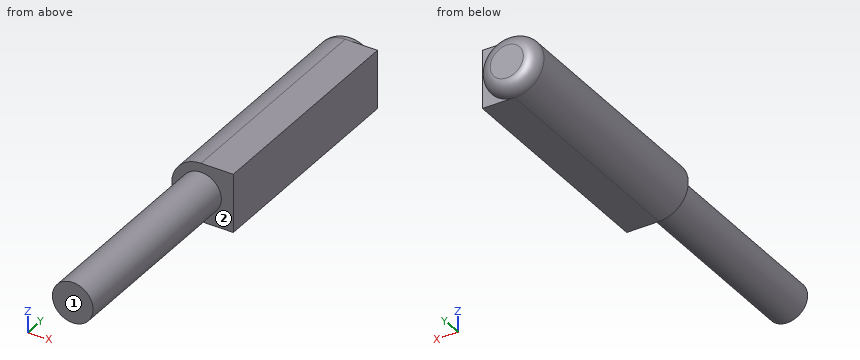
```python
from build123d import *

# Parameters (mm, degrees)
F0_R     = 11.5
F2_DEPTH = 95
F1_R     = 8
F3_DEPTH = 80
F4_R     = 5
F5_W     = 90
F5_H     = 23
F6_DEPTH = 12.7


with BuildPart() as f2:
    # F0 (on Front) → F2 (new body)
    with BuildSketch(Plane.XZ):
        Circle(F0_R)
    extrude(amount=-F2_DEPTH)

    # F1 (on Front) → F3 (join)
    with BuildSketch(Plane.XZ):
        Circle(F1_R)
    extrude(amount=F3_DEPTH)

    # F4
    f4_edges = [f2.edges().sort_by_distance(p)[0] for p in [
        (-11.5, 95, 0),
    ]]
    fillet(f4_edges, radius=F4_R)

    # F5 (on Right) → F6 (join)
    with BuildSketch(Plane.YZ):
        with Locations((45, 0)):
            Rectangle(F5_W, F5_H)
    extrude(amount=F6_DEPTH)


solid = f2.part
```
The listing builds one solid part. Answer for the finished solid, in the listing's coordinates (mm). Face numbers are marked on the shaded views. A direction names the side the tool comes from. Coordinates: 2 decimals unless noted, no trailing zeros. Loops run counter-clockwise (first coordinate to the right, second up) from the corner with the lowest first, then second, coordinate; pieces in that order, holes last. Notation, with made-up numbers: (45, -7) -> (99, -7) arc R25 cw to (99, 11) -> close; hole circle Ø3 at (24, 74). An arc over 180 degrees is marked (long way). Return JSON: item names as keys, results as strings. Group by question number.
(1) A cutting plane is placed at B-B on y = -24.5. Write down the section's boundary in (x, z), and give its area (3 significant figures).
(2) A cutting plane is placed at A-A on z = 0. Write down the section's boundary in (x, y), and give its area (3 significant figures).
(3) A cutting plane is placed at C-C on y = 74. Write down the section's boundary in (x, z).
(4) Which of the six approach directions +Z, -Z, +X, -X, +Y, -Y give full straight-line access (tool end or side, diameter ignored) to the marked faces 1 and 2?
(5) Given pin 1 Ø1.5 at (x, y) = (-7.5, -37.5) entering from +Z; pin 2 Ø1.5 at (x, z) = (7, 4.5) entering from +Y; pin 3 Ø1 at (x, y) = (-2.5, -44.5) entering from -Z, each flat-ended and moving along its own axis, determine where each tip first touches the part or whether it passes through.
(6) Find the intervals of material crossed by probe 1 along X at (y, z) = (52, 0.75); probe 2 along Z at (x, y) = (0.25, -31); probe 3 along Y at (x, z) = (11.5, 5.75), in increasing order. Write a range as from..to.
The answers:
{
 "1": {"outline": "circle Ø16 at (0, 0)", "area": "201 mm^2"},
 "2": {"outline": "(-11.5, 0) -> (-8, 0) -> (-8, -80) -> (8, -80) -> (8, 0) -> (12.7, 0) -> (12.7, 90) -> (11.5, 90) arc R5 ccw to (6.5, 95) -> (-6.5, 95) arc R5 ccw to (-11.5, 90) -> close", "area": "3,560 mm^2"},
 "3": {"outline": "(0, -11.5) -> (12.7, -11.5) -> (12.7, 11.5) -> (0, 11.5) arc R11.5 ccw to start"},
 "4": {"face 1": "+Z, -Z, +X, -X, -Y", "face 2": "-Y"},
 "5": {"pin 1": "stops at z = 4.29", "pin 2": "stops at y = 94.88", "pin 3": "stops at z = -7.75"},
 "6": {"probe 1": "x = -11.48..12.7", "probe 2": "z = -8..8", "probe 3": "y = 0..90"}
}
